Here's the drawing with two shaded views (mm, measured from the low corner). I have some questions. A direction names the side the tool comes from. Round coordinates to 2 decimals unless told otherwise and drop trailing zeros. Loops run counter-clockwise (first coordinate to the right, second up) from the corner with the lowest first, then second, coordinate; pieces in that order, holes last.
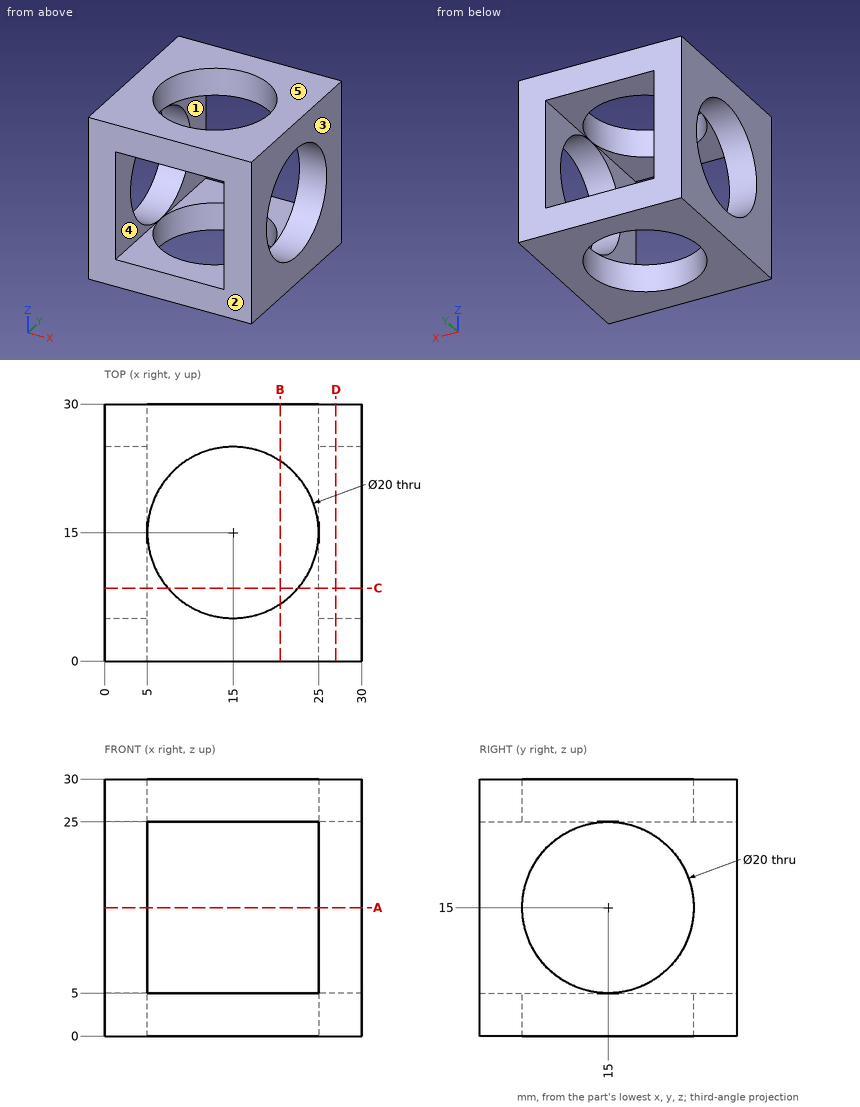
(1) Will this pin go through, and if not, where does the flat tip stop? P1, Ø12, axis at x = 15, y = 15, coming from the +Z side.
Worked answers:
P1: passes through
(2) If we section it at D-D, the plane x = 27: List the corners of the cut face in (y, z) for me, then the cut area to 3 significant figures.
Worked answers:
outline: (0, 0) - (30, 0) - (30, 30) - (0, 30) - close; hole circle Ø20 at (15, 15)
area: 586 mm2
(3) If we section it at C-C, the plane y = 8.5: List the corners of the cut face in (x, z) for me, then the cut area to 3 significant figures.
Worked answers:
outline: (0, 0) - (7.4, 0) - (7.4, 5) - (5, 5) - (5, 7.4) - (0, 7.4) - close; (0, 22.6) - (5, 22.6) - (5, 25) - (7.4, 25) - (7.4, 30) - (0, 30) - close; (22.6, 0) - (30, 0) - (30, 7.4) - (25, 7.4) - (25, 5) - (22.6, 5) - close; (22.6, 25) - (25, 25) - (25, 22.6) - (30, 22.6) - (30, 30) - (22.6, 30) - close
area: 196 mm2
(4) If we section it at B-B, the plane x = 20.5: List the corners of the cut face in (y, z) for me.
Worked answers:
outline: (0, 0) - (6.65, 0) - (6.65, 5) - (0, 5) - close; (0, 25) - (6.65, 25) - (6.65, 30) - (0, 30) - close; (23.35, 0) - (30, 0) - (30, 5) - (23.35, 5) - close; (23.35, 25) - (30, 25) - (30, 30) - (23.35, 30) - close
(5) If I drill on line 1 (Y direction, x = 28, z = 15), over which ranges is the centre line in solid material (lowest first)?
Worked answers:
line 1: y = 0 to 5, 25 to 30
(6) If we section it at A-A, the plane z = 15: List the corners of the cut face in (x, y) for me.
Worked answers:
outline: (0, 0) - (5, 0) - (5, 5) - (0, 5) - close; (0, 25) - (5, 25) - (5, 30) - (0, 30) - close; (25, 0) - (30, 0) - (30, 5) - (25, 5) - close; (25, 25) - (30, 25) - (30, 30) - (25, 30) - close
(7) For the marked faces 4 and 5, which set-ups out of +Z, -Z, +X, -X, +Y, -Y let a thin tool reach every point of the face, with its end or its side?
Worked answers:
face 4: +Y, -Y
face 5: +Z, +X, -X, +Y, -Y
(8) If we mould it in two halves opening along X, with no side actions, what happens to the marked faces 1, 2 and 3? For each: released by +X, released by -X, zero draft, split by the parting line, or undercut.
Worked answers:
face 1: undercut
face 2: zero draft
face 3: released by +X
